For this review, take the finished solid that the model builds, in its own axes (mm). A direction names the side the tool comes from. Round coordinates to 2 decimals unless told otherwise and drop trailing zeros. Loops run counter-clockwise (first coordinate to the right, second up) from the corner with the lowest first, then second, coordinate; pieces in that order, holes last.
1. Draft analysis for pull direction Y (two halves, no side actions). For faces 4 (the flat face through (63, 0, 2)), 5 (the flat face through (-2, 31.75, 2)), 6 (the flat face through (78, 31.75, 2)), state which applies: released by +Y, released by -Y, zero draft, split by the parting line, or undercut.
2. Consider section A-A on z = 2.55. State the section outline as (x, y) points (3 decimals), then the cut area to 3 significant figures.
3. To check wall thickness, follow line 1 along X through (y, z) = (2, 0.3) (3 decimals); line 2 along Y through (x, z) = (61.5, 1.7); line 3 along X through (y, z) = (30, 1.35) (3 decimals). State the ranges of each line that lie inside material, in increasing order.
4. Tool access review of faces 1 (the flat face through (47.625, -2, 2)), 2 (the flat face through (47.625, 46, 2)), 3 (the flat face through (76.2, 22, 2)): name each direction out of +Z, -Z, +X, -X, +Y, -Y from which nothing blocks a thin tool from reaching the whole face with its end or side.
5. Clearance check with flat-ended pins moving along their axes: pin 1 Ø1.6 at (x, z) = (19, 2) entering from -Y; pin 2 Ø1 at (x, z) = (-2, 2) entering from -Y; pin 3 Ø1.6 at (x, z) = (-2, 1.5) entering from +Y. State where each tip first meets the part, or that it passes through.
6. Consider section B-B on x = 73. State the section outline as (y, z) points (3 decimals), then the cut area to 3 significant figures.
7. Consider section C-C on y = 26.5. State the section outline as (x, z) points (3 decimals).
from build123d import *

# Parameters (mm, degrees)
SKETCH1_W           = 79.375
SKETCH1_H           = 44.45
BOSS_EXTRUDE1_DEPTH = 3.175
SKETCH2_W           = 3.175
SKETCH2_H           = 19.05
BOSS_EXTRUDE2_DEPTH = 3.175
SKETCH5_W           = 19.05
SKETCH5_H           = 3.175
BOSS_EXTRUDE3_DEPTH = 3.175
SKETCH3_W           = 3.175
SKETCH3_H           = 19.05
CUT_EXTRUDE1_DEPTH  = 3.175


with BuildPart() as part:
    # Sketch1 → Boss-Extrude1 (new body)
    with BuildSketch(Plane.XY):
        with Locations((39.6875, 22.225)):
            Rectangle(SKETCH1_W, SKETCH1_H)
    extrude(amount=BOSS_EXTRUDE1_DEPTH)

    # Sketch2 → Boss-Extrude2 (add)
    with BuildSketch(Plane.XY.offset(3.175)):
        with Locations((-1.5875, 22.225)):
            Rectangle(SKETCH2_W, SKETCH2_H)
    extrude(amount=-BOSS_EXTRUDE2_DEPTH)

    # Sketch5 → Boss-Extrude3 (add)
    with BuildSketch(Plane.XY.offset(3.175)):
        with Locations((38.1, 46.0375)):
            Rectangle(SKETCH5_W, SKETCH5_H)
        with Locations((38.1, -1.5875)):
            Rectangle(SKETCH5_W, SKETCH5_H)
    extrude(amount=-BOSS_EXTRUDE3_DEPTH)

    # Sketch3 → Cut-Extrude1 (cut)
    with BuildSketch(Plane.XY.offset(3.175)):
        with Locations((77.7875, 22.225)):
            Rectangle(SKETCH3_W, SKETCH3_H)
    extrude(amount=-CUT_EXTRUDE1_DEPTH, mode=Mode.SUBTRACT)


solid = part.part
Resolved:
1. face 4: released by -Y
1. face 5: released by +Y
1. face 6: undercut
2. outline: (-3.175, 12.7) - (0, 12.7) - (0, 0) - (28.575, 0) - (28.575, -3.175) - (47.625, -3.175) - (47.625, 0) - (79.375, 0) - (79.375, 12.7) - (76.2, 12.7) - (76.2, 31.75) - (79.375, 31.75) - (79.375, 44.45) - (47.625, 44.45) - (47.625, 47.625) - (28.575, 47.625) - (28.575, 44.45) - (0, 44.45) - (0, 31.75) - (-3.175, 31.75) - close
2. area: 3,650 mm2
3. line 1: x = 0 to 79.375
3. line 2: y = 0 to 44.45
3. line 3: x = -3.175 to 76.2
4. face 1: +Z, -Z, +X, -Y
4. face 2: +Z, -Z, +X, +Y
4. face 3: +Z, -Z, +X
5. pin 1: stops at y = 0
5. pin 2: stops at y = 12.7
5. pin 3: stops at y = 31.75
6. outline: (0, 0) - (44.45, 0) - (44.45, 3.175) - (0, 3.175) - close
6. area: 141 mm2
7. outline: (-3.175, 0) - (76.2, 0) - (76.2, 3.175) - (-3.175, 3.175) - close
